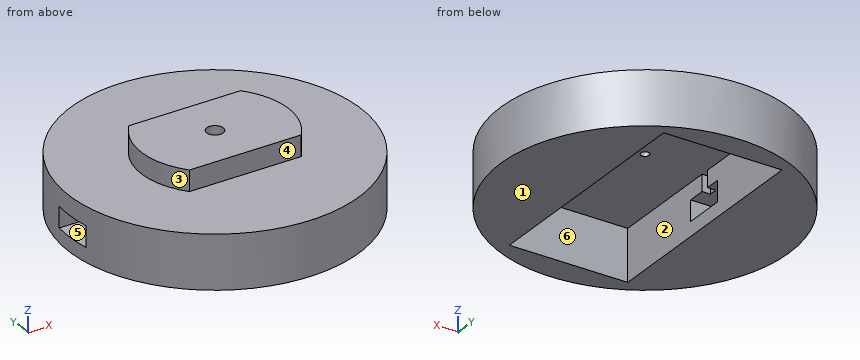
```python
from build123d import *

# Parameters (mm, degrees)
F0_R      = 35
F1_DEPTH  = 13
F3_DEPTH  = 12.5
F5_DEPTH  = 5
F6_R      = 2
F7_DEPTH  = 3
F8_R      = 1
F9_DEPTH  = 25
F10_W     = 10
F10_H     = 5
F11_DEPTH = 25
F12_W     = 1.986437419
F12_H     = 4.0204126202
F13_DEPTH = 2


with BuildPart() as f1:
    # F0 (on Top) → F1 (new body)
    with BuildSketch(Plane.XY):
        Circle(F0_R)
    extrude(amount=F1_DEPTH)

    # F2 (on face) → F3 (cut)
    with BuildSketch(Plane(origin=(0, 0, 0), x_dir=(1, 0, 0), z_dir=(0, 0, -1))):
        Polygon((14.4, 28.3542412236), (-14.4, 28.3542412236), (-14.4, 0), (0, 0), (14.4, 0), align=None)
        Polygon((0, 0), (-14.4, 0), (-14.4, -28.8457587764), (14.4, -28.8457587764), (14.4, 0), align=None)
    extrude(amount=-F3_DEPTH, mode=Mode.SUBTRACT)

    # F4 (on face) → F5 (join)
    with BuildSketch(Plane.XY.offset(13)):
        with BuildLine():
            ThreePointArc((13.6, -11.25), (16.6066628195, -5.978398615), (17.65, 0))
            ThreePointArc((17.65, 0), (16.6066628195, 5.978398615), (13.6, 11.25))
            Line((13.6, 11.25), (-13.6, 11.25))
            ThreePointArc((-13.6, 11.25), (-17.65, 0), (-13.6, -11.25))
            Line((-13.6, -11.25), (0, -11.25))
            Line((0, -11.25), (13.6, -11.25))
        make_face()
    extrude(amount=F5_DEPTH)

    # F6 (on face) → F7 (cut)
    with BuildSketch(Plane.XY.offset(18)):
        Circle(F6_R)
    extrude(amount=-F7_DEPTH, mode=Mode.SUBTRACT)

    # F8 (on face) → F9 (cut)
    with BuildSketch(Plane.XY.offset(15)):
        Circle(F8_R)
    extrude(amount=-F9_DEPTH, mode=Mode.SUBTRACT)

    # F10 (on face) → F11 (cut)
    with BuildSketch(Plane.YZ.offset(-14.4)):
        with Locations((-0.0396446604, 5.9795873798)):
            Rectangle(F10_W, F10_H)
    extrude(amount=-F11_DEPTH, mode=Mode.SUBTRACT)

    # F12 (on face) → F13 (cut)
    with BuildSketch(Plane.YZ.offset(-14.4)):
        with Locations((0.2311340359, 10.4897936899)):
            Rectangle(F12_W, F12_H)
    extrude(amount=-F13_DEPTH, mode=Mode.SUBTRACT)


solid = f1.part
```
Verification items for the finished model (mm, model axes). Face numbers are marked on the shaded views. A direction names the side the tool comes from. Coordinates: 2 decimals unless noted, no trailing zeros. Loops run counter-clockwise (first coordinate to the right, second up) from the corner with the lowest first, then second, coordinate; pieces in that order, holes last. Notation, with made-up numbers: (31, 19.5) - (66, 19.5) arc R21 cw to (66, 55.5) - close; hole circle Ø6 at (-36.75, -31.5). An arc over 180 degrees is marked (long way). Put each result on its own line as item: value.
Item 1: Set-up check for the marked faces 4, 5 and 6: record each of +Z, -Z, +X, -X, +Y, -Y from which the full face is reachable in a straight line by a thin tool's end or side.
Conclusion:
face 4: +Z, +X, -X, -Y
face 5: -X
face 6: -Z
Item 2: Scan lines: line 1 along Y through (x, z) = (0, 16.1); line 2 along Z through (x, y) = (-16.5, 1); line 3 along Y through (x, z) = (0, 14.45). Record each from-to range of solid material in increasing order.
Conclusion:
line 1: y = -11.25 to -2, 2 to 11.25
line 2: z = 0 to 3.48, 8.48 to 18
line 3: y = -11.25 to -1, 1 to 11.25
Item 3: Gauge pin test, flat ends, axial feed: pin 1 Ø6 at (x, z) = (-1.5, 5.5) entering from -Y; pin 2 Ø15.5 at (x, y) = (-4, -2.5) entering from -Z; pin 3 Ø5.5 at (x, z) = (-20.5, 5) entering from -Y. Record the tip position at first contact, or that the pin passes through.
Conclusion:
pin 1: stops at y = -35
pin 2: stops at z = 12.5
pin 3: stops at y = -30.17
Item 4: Draft check along X on the marked faces 1, 2 and 3. Enter one of: pulls with the +X half, pulls with the -X half, needs draft (parallel to the pull), parting line crosses it, or undercut.
Conclusion:
face 1: needs draft
face 2: undercut
face 3: pulls with the -X half
Item 5: Section check D-D (x = -28). Enter the section's corners in (y, z), then the cut area to 3 significant figures.
Conclusion:
outline: (-21, 0) - (21, 0) - (21, 13) - (-21, 13) - close; hole (-5.04, 3.48) - (4.96, 3.48) - (4.96, 8.48) - (-5.04, 8.48) - close
area: 496 mm2
Item 6: Section check A-A (x = 0). Enter the section's corners in (y, z), then the cut area to 4 significant figures.
Conclusion:
outline: (-35, 0) - (-28.35, 0) - (-28.35, 12.5) - (-1, 12.5) - (-1, 15) - (-2, 15) - (-2, 18) - (-11.25, 18) - (-11.25, 13) - (-35, 13) - close; (1, 12.5) - (28.85, 12.5) - (28.85, 0) - (35, 0) - (35, 13) - (11.25, 13) - (11.25, 18) - (2, 18) - (2, 15) - (1, 15) - close
area: 290.5 mm2
Item 7: Section check B-B (y = -3). Enter the section's corners in (x, z).
Conclusion:
outline: (-34.87, 0) - (-14.4, 0) - (-14.4, 3.48) - (-34.87, 3.48) - close; (-34.87, 8.48) - (-14.4, 8.48) - (-14.4, 12.5) - (14.4, 12.5) - (14.4, 0) - (34.87, 0) - (34.87, 13) - (17.39, 13) - (17.39, 18) - (-17.39, 18) - (-17.39, 13) - (-34.87, 13) - close
Item 8: Section check C-C (z = 11). Enter the section's corners in (x, y), then the cut area to 3 significant figures.
Conclusion:
outline: circle Ø70 at (0, 0); hole (-16.4, -0.76) - (-14.4, -0.76) - (-14.4, -28.35) - (14.4, -28.35) - (14.4, 28.85) - (-14.4, 28.85) - (-14.4, 1.22) - (-16.4, 1.22) - close
area: 2,200 mm2
